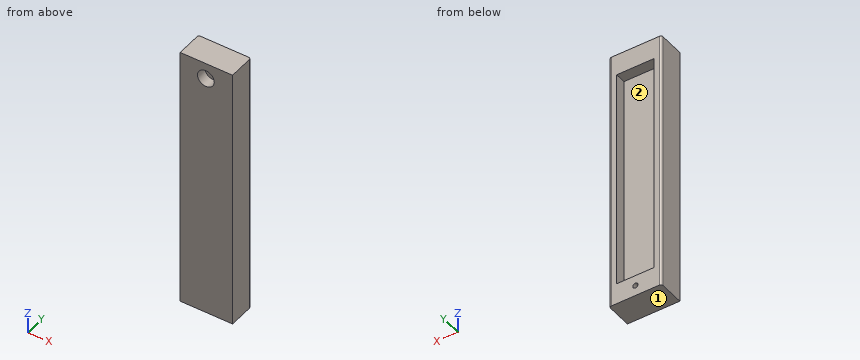
```python
from build123d import *

# Parameters (mm, degrees)
SKETCH1_W               = 49
SKETCH1_H               = 20
BOSS_EXTRUDE1_DEPTH     = 125
SKETCH3_W               = 49
SKETCH3_H               = 250
BOSS_EXTRUDE2_DEPTH     = 5
CUT_EXTRUDE1_DEPTH      = 130.808512818
CUT_EXTRUDE1_DEPTH_BACK = 10
SKETCH2_R               = 2.4
SKETCH5_W               = 35
SKETCH5_H               = 210
CUT_EXTRUDE3_DEPTH      = 10
FILLET1_R               = 2
SKETCH4_R               = 7.874
CUT_EXTRUDE2_DEPTH      = 10


with BuildPart() as part:
    # Sketch1 → Boss-Extrude1 (new, symmetric)
    with BuildSketch(Plane.XY):
        Rectangle(SKETCH1_W, SKETCH1_H)
    extrude(amount=BOSS_EXTRUDE1_DEPTH, both=True)

    # Sketch3 → Boss-Extrude2 (add)
    with BuildSketch(Plane(origin=(0, 10, 0), x_dir=(1, 0, 0), z_dir=(0, 1, 0))):
        Rectangle(SKETCH3_W, SKETCH3_H)
    extrude(amount=BOSS_EXTRUDE2_DEPTH)

    # Sketch2 → Cut-Extrude1 (cut, two sides: drawn at the far end of the back side and taken through both)
    with BuildSketch(Plane(origin=(0, 15, 0), x_dir=(1, 0, 0), z_dir=(0, 1, 0)).offset(-CUT_EXTRUDE1_DEPTH_BACK)):
        with Locations(Location((0, 115, 0), (0, 0, 90))):
            Circle(SKETCH2_R)
    extrude(amount=CUT_EXTRUDE1_DEPTH + CUT_EXTRUDE1_DEPTH_BACK, mode=Mode.SUBTRACT)

    # Sketch5 → Cut-Extrude3 (cut)
    with BuildSketch(Plane(origin=(0, 15, 0), x_dir=(1, 0, 0), z_dir=(0, 1, 0))):
        Rectangle(SKETCH5_W, SKETCH5_H)
    extrude(amount=-CUT_EXTRUDE3_DEPTH, mode=Mode.SUBTRACT)

    # Fillet1
    fillet1_edges = [part.edges().sort_by_distance(p)[0] for p in [
        (-24.5, 15, 0),
        (24.5, 15, 0),
    ]]
    fillet(fillet1_edges, radius=FILLET1_R)

    # Sketch4 → Cut-Extrude2 (cut)
    with BuildSketch(Plane.XZ.offset(10)):
        with Locations(Location((-0.5, 110, 0), (0, 0, 270))):
            Circle(SKETCH4_R)
    extrude(amount=-CUT_EXTRUDE2_DEPTH, mode=Mode.SUBTRACT)


solid = part.part
```
Can you work these out from the model? Positions are in its coordinate system, mm. Face numbers are marked on the shaded views. A direction names the side the tool comes from. Round coordinates to 2 decimals unless told otherwise and drop trailing zeros. Loops run counter-clockwise (first coordinate to the right, second up) from the corner with the lowest first, then second, coordinate; pieces in that order, holes last. Notation, with made-up numbers: (53.25, 81) -> (59.25, 81) arc R22 cw to (59.25, 89) -> close; hole circle Ø9 at (48.25, -35). An arc over 180 degrees is marked (long way). Answer in a Markdown table with one row per item.
Item 1: Will these pins go through, and if not, where does the flat tip stop? P1, Ø8, axis at x = 1.5, z = 110, coming from the -Y side; P2, Ø17.5, axis at x = -8, z = -39.5, coming from the +Y side.
Answer block:
| item | result |
|---|---|
| P1 | y = 0 |
| P2 | y = 5 |
Item 2: Suppose I cut it at C-C, the plane y = 9. List the corners of the cut face in (x, z) for me.
Answer block:
| item | result |
|---|---|
| outline | (-24.5, -125) -> (24.5, -125) -> (24.5, 125) -> (-24.5, 125) -> close; hole (-17.5, -105) -> (17.5, -105) -> (17.5, 105) -> (-17.5, 105) -> close; hole circle Ø4.8 at (0, -115) |
Item 3: Suppose I cut it at A-A, the plane z = 110. List the corners of the cut face in (x, y) for me.
Answer block:
| item | result |
|---|---|
| outline | (-24.5, -10) -> (-8.37, -10) -> (-8.37, 0) -> (7.37, 0) -> (7.37, -10) -> (24.5, -10) -> (24.5, 13) arc R2 ccw to (22.5, 15) -> (-22.5, 15) arc R2 ccw to (-24.5, 13) -> close |
Item 4: On a 3-axis mill with a long thin cutter (end or side, diameter ignored), from which of +Z, -Z, +X, -X, +Y, -Y can I reach the whole of each face in a straight line? I mean the marked faces 1 and 2. Say none if no direction works.
Answer block:
| item | result |
|---|---|
| face 1 | -Z, +X, -X, +Y, -Y |
| face 2 | +Y |
Item 5: Suppose I cut it at D-D, the plane z = 54.5. List the corners of the cut face in (x, y) for me.
Answer block:
| item | result |
|---|---|
| outline | (-24.5, -10) -> (24.5, -10) -> (24.5, 13) arc R2 ccw to (22.5, 15) -> (17.5, 15) -> (17.5, 5) -> (-17.5, 5) -> (-17.5, 15) -> (-22.5, 15) arc R2 ccw to (-24.5, 13) -> close |
Item 6: Suppose I cut it at B-B, the plane y = -3. List the corners of the cut face in (x, z) for me, plus the area to 3 significant figures.
Answer block:
| item | result |
|---|---|
| outline | (-24.5, -125) -> (24.5, -125) -> (24.5, 125) -> (-24.5, 125) -> close; hole circle Ø15.75 at (-0.5, 110) |
| area | 12,100 mm² |
Item 7: If I drill on probe 1 along X at (y, z) = (7.5, -82.5); probe 2 along Z at (x, y) = (-9, 13.5); probe 3 along X at (y, z) = (-4.5, 110), over which ranges is the centre line in solid material (lowest first)?
Answer block:
| item | result |
|---|---|
| probe 1 | -24.5 to -17.5, 17.5 to 24.5 |
| probe 2 | -125 to -105, 105 to 125 |
| probe 3 | -24.5 to -8.37, 7.37 to 24.5 |
